Check sheet for the modelled part. Datum: model origin and axes. Units: mm. A direction names the side the tool comes from. Give positions to 0.01 mm unless a question says otherwise; leave off trailing zeros. Order: outer loops, then holes, each group sorted by start corner. A loop starts at its lowest first (then second) coordinate and runs counter-clockwise, first axis right, second up.
Item 1: Sectioned sample at B-B on z = -72. Record the boundary of the cut face in (x, y).
Item 2: Gauge pin test, flat ends, axial feed: P1, Ø3, axis at y = 6.5, z = -93, coming from the -X side; P2, Ø5, axis at x = 105.5, y = 5.5, coming from the -Z side; P3, Ø5, axis at x = 14.5, z = -85, coming from the +Y side. Record the tip position at first contact, or that the pin passes through.
Item 3: Sectioned sample at A-A on x = 115. Record the boundary of the cut face in (y, z), and give its area (3 significant figures).
Item 4: Sectioned sample at D-D on x = -121. Record the boundary of the cut face in (y, z), and give its area (3 significant figures).
Item 5: Access from +Z, -Z, +X, -X, +Y, -Y to the whole of each face (thin tool, end or side, straight path). Record for faces 4 (the flat face through (-110, 5, -20)), 5 (the flat face through (-2, 10, -105)), 6 (the flat face through (60, 3, -25)), 7 (the flat face through (113, 3, -25)), 8 (the flat face through (-2, 2.8, 0)).
Item 6: Material ranges on line 1 along Y through (x, z) = (121, -42.5); line 2 along Z through (x, y) = (-106, 4.25); line 3 along X through (y, z) = (7.75, -109), recorded low to high.
Item 7: Sectioned sample at C-C on y = 5. Count the separate pieces of the cut face and the enclosed holes in it, and give its area (3 significant figures).
Item 8: Release check for a two-part mould opening along X. For faces 1 (the flat face through (-2, 0, -70)), 2 (the flat face through (-105, 5, -110.5)), 3 (the flat face through (-133.78, 4.93, -70.16)) record: released by +X, released by -X, zero draft, split by the parting line, or undercut.
from build123d import *

# Parameters (mm, degrees)
SKETCH_1_W          = 250
SKETCH_1_H          = 125
EXTRUDE_1_DEPTH     = 10
SKETCH_5_W          = 10
SKETCH_5_H          = 10
CUT_EXTRUDE_1_DEPTH = 10
CUT_EXTRUDE_2_DEPTH = 3
SKETCH_7_W          = 30
SKETCH_7_H          = 4
CUT_EXTRUDE_3_DEPTH = 50
EXTRUDE_3_DEPTH     = 250
EXTRUDE_4_REACH     = 191.684
SKETCH_11_W         = 10.5
SKETCH_11_H         = 10.5
SKETCH_11_H_2       = 10.520913438
SKETCH_11_W_2       = 10.415866522
CUT_EXTRUDE_4_DEPTH = 202.519860157


with BuildPart() as part:
    # 草图1 → 凸台-拉伸1 (new body)
    with BuildSketch(Plane(origin=(0, 0, 0), x_dir=(1, 0, 0), z_dir=(0, 1, 0))):
        with Locations((0, 62.5)):
            Rectangle(SKETCH_1_W, SKETCH_1_H)
    extrude(amount=EXTRUDE_1_DEPTH)

    # 草图5 → 切除-拉伸1 (cut)
    with BuildSketch(Plane(origin=(0, 10, 0), x_dir=(1, 0, 0), z_dir=(0, 1, 0))):
        with Locations((-105, 105)):
            Rectangle(SKETCH_5_W, SKETCH_5_H)
        with Locations((-105, 20)):
            Rectangle(SKETCH_5_W, SKETCH_5_H)
        with Locations((105, 105)):
            Rectangle(SKETCH_5_W, SKETCH_5_H)
        with Locations((105, 20)):
            Rectangle(SKETCH_5_W, SKETCH_5_H)
    extrude(amount=-CUT_EXTRUDE_1_DEPTH, mode=Mode.SUBTRACT)

    # 草图6 → 切除-拉伸2 (cut)
    with BuildSketch(Plane(origin=(0, 10, 0), x_dir=(1, 0, 0), z_dir=(0, 1, 0))):
        with BuildLine():
            Line((-100, 0), (100, 0))
            ThreePointArc((100, 0), (0, 100), (-100, 0))
        make_face()
    extrude(amount=-CUT_EXTRUDE_2_DEPTH, mode=Mode.SUBTRACT)

    # 草图7 → 切除-拉伸3 (cut)
    with BuildSketch(Plane.XY):
        with Locations((-90, 5)):
            Rectangle(SKETCH_7_W, SKETCH_7_H)
        with Locations((-40, 5)):
            Rectangle(SKETCH_7_W, SKETCH_7_H)
        with Locations((10, 5)):
            Rectangle(SKETCH_7_W, SKETCH_7_H)
        with Locations((60, 5)):
            Rectangle(SKETCH_7_W, SKETCH_7_H)
        with Locations((110, 5)):
            Rectangle(SKETCH_7_W, SKETCH_7_H)
    extrude(amount=-CUT_EXTRUDE_3_DEPTH, mode=Mode.SUBTRACT)

    # 草图8 → 凸台-拉伸3 (add)
    with BuildSketch(Plane.ZY.offset(125)):
        Polygon((-125, 10), (-125, 0), (-142.320508076, 0), align=None)
    extrude(amount=-EXTRUDE_3_DEPTH)

    # 凸台-拉伸4: up to this plane
    extrude_4_end = Plane(origin=(145, 0, -142.320508076), z_dir=(0, 0.8660254037844419, -0.4999999999999944))
    # 草图9 → 凸台-拉伸4 (add, up to the surface)
    with BuildSketch(Plane.XY, mode=Mode.PRIVATE) as extrude_4_sk1:
        Polygon((-125, 10), (-125, 0), (-142.320508076, 0), align=None)
    extrude_4_tool1 = split(extrude(extrude_4_sk1.sketch, amount=-EXTRUDE_4_REACH, mode=Mode.PRIVATE), bisect_by=extrude_4_end, keep=Keep.BOTH, mode=Mode.PRIVATE)
    add(extrude_4_tool1.solids().sort_by_distance((-130.773503, 3.333333, 0))[0])
    # 草图9 → 凸台-拉伸4 (add, up to the surface)
    with BuildSketch(Plane.XY, mode=Mode.PRIVATE) as extrude_4_sk2:
        Polygon((125, 10), (125, 0), (142.320508076, 0), align=None)
    extrude_4_tool2 = split(extrude(extrude_4_sk2.sketch, amount=-EXTRUDE_4_REACH, mode=Mode.PRIVATE), bisect_by=extrude_4_end, keep=Keep.BOTH, mode=Mode.PRIVATE)
    add(extrude_4_tool2.solids().sort_by_distance((130.773503, 3.333333, 0))[0])

    # 草图11 → 切除-拉伸4 (cut, through all)
    with BuildSketch(Plane(origin=(0, 10, 0), x_dir=(1, 0, 0), z_dir=(0, 1, 0))):
        with Locations((-104.75, 105.25)):
            Rectangle(SKETCH_11_W, SKETCH_11_H)
        with Locations((-104.75, 20.260456719)):
            Rectangle(SKETCH_11_W, SKETCH_11_H_2)
        with Locations((105.207933261, 20.260456719)):
            Rectangle(SKETCH_11_W_2, SKETCH_11_H_2)
        with Locations((105.207933261, 105.25)):
            Rectangle(SKETCH_11_W_2, SKETCH_11_H)
    extrude(amount=-CUT_EXTRUDE_4_DEPTH, mode=Mode.SUBTRACT)


solid = part.part
Report:
1. outline: (-142.32, 0) - (142.32, 0) - (125, 10) - (69.4, 10) - (69.4, 7) - (-69.4, 7) - (-69.4, 10) - (-125, 10) - close
2. P1: stops at x = -133.66
2. P2: stops at z = -137.12
2. P3: stops at y = 7
3. outline: (0, -142.32) - (10, -125) - (10, 0) - (7, 0) - (7, -50) - (3, -50) - (3, 0) - (0, 0) - close
3. area: 1,140 mm2
4. outline: (0, -142.32) - (10, -125) - (10, 0) - (0, 0) - close
4. area: 1,340 mm2
5. face 4: +Y, -Y
5. face 5: +Z, -Z, +X, -X, +Y
5. face 6: +Z, +Y
5. face 7: +Z
5. face 8: +Z, +X, -X, +Y, -Y
6. line 1: y = 0 to 3, 7 to 10
6. line 2: z = -134.96 to -110.5, -100 to -25.52, -15 to 0
6. line 3: x = -128.9 to -110, -99.5 to 100, 110.42 to 128.9
7. separate pieces: 1
7. enclosed holes: 2
7. area: 28,000 mm2
8. face 1: zero draft
8. face 2: undercut
8. face 3: released by -X
